```python
from build123d import *

# Parameters (mm, degrees)
F0_W     = 5.98
F0_H     = 31.77
F1_DEPTH = 9.5
F3_D     = 5
F4_R     = 2.445
F5_DEPTH = 2.69
F6_W     = 2.92
F6_H     = 28.9
F7_DEPTH = 2.78
F9_DEPTH = 2.75


with BuildPart() as f1:
    # F0 (on Front) → F1 (new body)
    with BuildSketch(Plane.XZ):
        with Locations((-21.5895947321, 10.6426752984)):
            Rectangle(F0_W, F0_H)
    extrude(amount=F1_DEPTH)

    # F3 (through all)
    with Locations(Plane.YZ):
        with Locations((-4.02, 19.2140168432), (-4.02, 12.1440168432), (-4.02, 5.0740168432)):
            Hole(F3_D / 2)

    # F4 (on Front) → F5 (join)
    with BuildSketch(Plane.XZ):
        with Locations((-21.4179256038, 22.0790577062)):
            Circle(F4_R)
        with Locations((-21.4179256038, 14.3290577062)):
            Circle(F4_R)
        with Locations((-21.4179256038, 6.5790577062)):
            Circle(F4_R)
        with Locations((-21.4179256038, -1.1709422938)):
            Circle(F4_R)
    extrude(amount=-F5_DEPTH)

    # F6 (on face) → F7 (cut)
    with BuildSketch(Plane.XZ.offset(9.5)):
        with Locations((-21.5895947321, 10.5476752984)):
            Rectangle(F6_W, F6_H)
    extrude(amount=-F7_DEPTH, mode=Mode.SUBTRACT)

    # F8 (on face) → F9 (join)
    with BuildSketch(Plane.XZ.offset(6.72)):
        with BuildLine():
            ThreePointArc((-23.0495947321, 18.4560718795), (-21.345700419, 17.5789010333), (-20.1375805098, 19.0665605403))
            ThreePointArc((-20.1375805098, 19.0665605403), (-21.345700419, 20.5542200474), (-23.0495947321, 19.6770492011))
            Line((-23.0495947321, 19.6770492011), (-23.0495947321, 18.4560718795))
        make_face()
        with BuildLine():
            ThreePointArc((-20.1375805098, 11.0265605403), (-21.345700419, 12.5142200474), (-23.0495947321, 11.6370492011))
            Line((-23.0495947321, 11.6370492011), (-23.0495947321, 10.4160718795))
            ThreePointArc((-23.0495947321, 10.4160718795), (-21.345700419, 9.5389010333), (-20.1375805098, 11.0265605403))
        make_face()
        with BuildLine():
            Line((-23.0495947321, 2.3760718795), (-23.0495947321, 3.5970492011))
            ThreePointArc((-23.0495947321, 3.5970492011), (-23.1775805098, 2.9865605403), (-23.0495947321, 2.3760718795))
        make_face()
        with BuildLine():
            ThreePointArc((-20.1375805098, 2.9865605403), (-21.345700419, 4.4742200474), (-23.0495947321, 3.5970492011))
            Line((-23.0495947321, 3.5970492011), (-23.0495947321, 2.3760718795))
            ThreePointArc((-23.0495947321, 2.3760718795), (-21.345700419, 1.4989010333), (-20.1375805098, 2.9865605403))
        make_face()
    extrude(amount=F9_DEPTH)


solid = f1.part
```
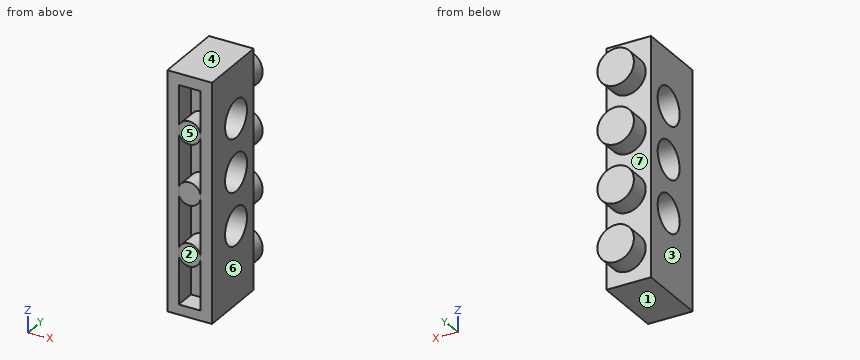
Geometry check sheet. Reference: the model listing, model coordinates, mm. Face numbers are marked on the shaded views. A direction names the side the tool comes from. Round coordinates to 2 decimals unless told otherwise and drop trailing zeros. Loops run counter-clockwise (first coordinate to the right, second up) from the corner with the lowest first, then second, coordinate; pieces in that order, holes last. Notation, with made-up numbers: (75, -28.5) - (119, -28.5) arc R9 ccw to (119, -19.5) - close; hole circle Ø8 at (1, 83.25). An arc over 180 degrees is marked (long way). Write item = value, one per line. Start each with the question number.
1. Section check B-B on x = -19.8. Enter the section's corners in (y, z).
2. Section check C-C on z = 16. Enter the section's corners in (x, y), then the cut area to 3 significant figures.
3. Section check D-D on z = 23. Enter the section's corners in (x, y).
4. Thickness scan on line 1 (Z direction, x = -22.05, y = -4.02); line 2 (Z direction, x = -21.55, y = -8.25); line 3 (Y direction, x = -21.9, z = 5). Record the ranges inside material, lowest first.
5. Depth check by flat-ended pin: pin 1 (1.5 mm diameter, centred on x = -21, z = 3.5, fed in from -Y). Enter the tip coordinate at first touch or a pass-through.
6. Section check A-A on y = -4.02. Enter the section's corners in (x, z).
7. Set-up check for the marked faces 5, 6 and 7: record each of +Z, -Z, +X, -X, +Y, -Y from which the full face is reachable in a straight line by a thin tool's end or side.
8. Mould release check, pull along Z, two halves, no side actions. Record for the marked faces 1, 2, 3 and 4: released by +Z, released by -Z, zero draft, split by the parting line, or undercut.
Working result:
q1.outline = (-9.5, -5.24) - (0, -5.24) - (0, -3) - (2.69, -3) - (2.69, 0.66) - (0, 0.66) - (0, 4.75) - (2.69, 4.75) - (2.69, 8.41) - (0, 8.41) - (0, 12.5) - (2.69, 12.5) - (2.69, 16.16) - (0, 16.16) - (0, 20.25) - (2.69, 20.25) - (2.69, 23.91) - (0, 23.91) - (0, 26.53) - (-9.5, 26.53) - close; hole circle Ø5 at (-4.02, 5.07); hole circle Ø5 at (-4.02, 12.14); hole circle Ø5 at (-4.02, 19.21)
q2.outline = (-24.58, -9.5) - (-23.05, -9.5) - (-23.05, -6.72) - (-20.13, -6.72) - (-20.13, -9.5) - (-18.6, -9.5) - (-18.6, 0) - (-19.63, 0) - (-19.63, 2.69) - (-23.2, 2.69) - (-23.2, 0) - (-24.58, 0) - close
q2.area = 58.3 mm^2
q3.outline = (-24.58, -9.5) - (-23.05, -9.5) - (-23.05, -6.72) - (-20.13, -6.72) - (-20.13, -9.5) - (-18.6, -9.5) - (-18.6, 0) - (-19.15, 0) - (-19.15, 2.69) - (-23.68, 2.69) - (-23.68, 0) - (-24.58, 0) - close
q4.line_1 = -5.24 to 2.57, 7.57 to 9.64, 14.64 to 16.71, 21.71 to 26.53
q4.line_2 = -5.24 to -3.9, 1.47 to 4.5, 9.51 to 12.54, 17.55 to 20.58, 25 to 26.53
q4.line_3 = -6.72 to -6.52, -1.52 to 2.69
q5.pin_1 = -9.47
q6.outline = (-24.58, -5.24) - (-18.6, -5.24) - (-18.6, 2.57) - (-24.58, 2.57) - close; (-24.58, 7.57) - (-18.6, 7.57) - (-18.6, 9.64) - (-24.58, 9.64) - close; (-24.58, 14.64) - (-18.6, 14.64) - (-18.6, 16.71) - (-24.58, 16.71) - close; (-24.58, 21.71) - (-18.6, 21.71) - (-18.6, 26.53) - (-24.58, 26.53) - close
q7.face_5 = -Y
q7.face_6 = +Z, -Z, +X, +Y, -Y
q7.face_7 = +Y
q8.face_1 = released by -Z
q8.face_2 = undercut
q8.face_3 = zero draft
q8.face_4 = released by +Z
